Verification items for the finished model (mm, model axes). Face numbers are marked on the shaded views. A direction names the side the tool comes from. Give positions to 0.01 mm unless a question says otherwise; leave off trailing zeros. Loops run counter-clockwise (first coordinate to the right, second up) from the corner with the lowest first, then second, coordinate; pieces in that order, holes last. Notation, with made-up numbers: (16, -32) - (72, -32) arc R5 cw to (72, -25) - close; hole circle Ø4 at (4, 14.5). An arc over 180 degrees is marked (long way). One line per question, with ' | ' between items. Start each with the question number.
1. Thickness scan on line 1 along Y through (x, z) = (24, 34); line 2 along X through (y, z) = (109.25, 5); line 3 along Y through (x, z) = (4, 23.5). Record the ranges inside material, lowest first. Write a range as from..to.
2. Section check A-A, the plane z = 19.5. State how many separate pieces and enclosed holes the cut face has, then the cut area to 3 significant figures.
3. Depth check by flat-ended pin: pin 1 Ø6.5 at (x, y) = (58, 3) entering from -Z; pin 2 Ø10 at (x, y) = (10.5, 77) entering from -Z; pin 3 Ø1.3 at (x, y) = (59, 109) entering from +Z; pin 4 Ø2 at (x, y) = (46.5, 67) entering from +Z. Enter the tip coordinate at first touch or a pass-through.
4. Tool access check on the marked faces 5, 6 and 7. Record the directions out of +Z, -Z, +X, -X, +Y, -Y that give a thin tool (end or side, any length) a straight path to the whole face; none if there is none.
5. Mould release check, pull along X, two halves, no side actions. Record for the marked faces 1, 2, 3 and 4: +X half, -X half, draft (parallel to the pull), parting line (faces both ways), or undercut.
6. Section check B-B, the plane y = 28. Enter the section's corners in (x, z), then the cut area to 3 significant figures.
7. Section check C-C, the plane z = 9. Enter the section's corners in (x, y).
8. Section check D-D, the plane y = 63.5. Enter the section's corners in (x, z), then the cut area to 3 significant figures.
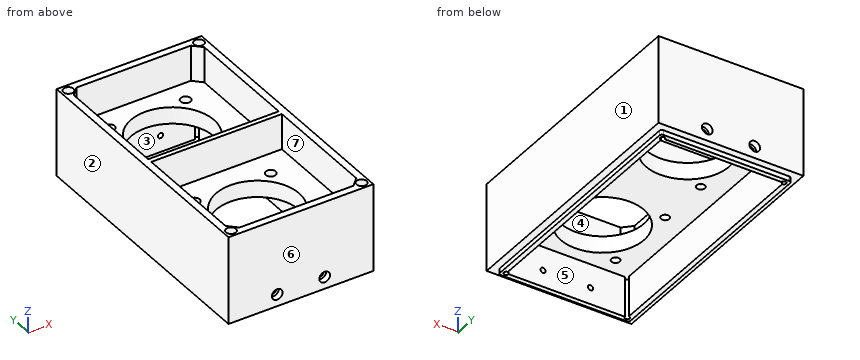
from build123d import *

# Parameters (mm, degrees)
SKETCH1_W           = 61
SKETCH1_H           = 111
SKETCH1_W_2         = 51
SKETCH1_H_2         = 101
BOSS_EXTRUDE1_DEPTH = 15
SKETCH2_W           = 61
SKETCH2_H           = 111
BOSS_EXTRUDE2_DEPTH = 7
SKETCH3_R           = 17.5
SKETCH3_R_2         = 1.75
CUT_EXTRUDE1_DEPTH  = 23
SKETCH4_R           = 2.1
CUT_EXTRUDE2_DEPTH  = 5
SKETCH5_W           = 55
SKETCH5_H           = 105
SKETCH5_W_2         = 51
SKETCH5_H_2         = 101
BOSS_EXTRUDE3_DEPTH = 2
FILLET1_R           = 1
SKETCH6_R           = 1.1
CUT_EXTRUDE3_DEPTH  = 112
SKETCH7_R           = 2.25
CUT_EXTRUDE4_DEPTH  = 2.5
SKETCH8_R           = 2.25
CUT_EXTRUDE5_DEPTH  = 2.5
CUT_EXTRUDE6_START  = -17
SKETCH9_R           = 1
CUT_EXTRUDE6_DEPTH  = 17
SKETCH10_W          = 61
SKETCH10_H          = 111
SKETCH10_W_2        = 55
SKETCH10_H_2        = 105
SKETCH10_H_3        = 2
BOSS_EXTRUDE4_DEPTH = 15
SKETCH11_R          = 2.1
CUT_EXTRUDE7_DEPTH  = 6


with BuildPart() as part:
    # Sketch1 → Boss-Extrude1 (new body)
    with BuildSketch(Plane.XY):
        with Locations((30.5, 55.5)):
            Rectangle(SKETCH1_W, SKETCH1_H)
        with Locations((30.5, 55.5)):
            Rectangle(SKETCH1_W_2, SKETCH1_H_2, mode=Mode.SUBTRACT)
    extrude(amount=BOSS_EXTRUDE1_DEPTH)

    # Sketch2 → Boss-Extrude2 (add)
    with BuildSketch(Plane.XY.offset(15)):
        with Locations((30.5, 55.5)):
            Rectangle(SKETCH2_W, SKETCH2_H)
    extrude(amount=BOSS_EXTRUDE2_DEPTH)

    # Sketch3 → Cut-Extrude1 (cut, through all)
    with BuildSketch(Plane.XY.offset(22)):
        with Locations((30.5, 83)):
            Circle(SKETCH3_R)
        with Locations((30.5, 28)):
            Circle(SKETCH3_R)
        with BuildLine():
            ThreePointArc((46.5, 13.75), (45.262563133, 13.237436867), (44.75, 12))
            Line((44.75, 12), (46.5, 12))
            Line((46.5, 12), (46.5, 13.75))
        make_face()
        with BuildLine():
            Line((46.5, 12), (44.75, 12))
            ThreePointArc((44.75, 12), (46.5, 10.25), (48.25, 12))
            ThreePointArc((48.25, 12), (47.737436867, 13.237436867), (46.5, 13.75))
            Line((46.5, 13.75), (46.5, 12))
        make_face()
        with Locations((46.5, 99)):
            Circle(SKETCH3_R_2)
        with Locations((14.5, 99)):
            Circle(SKETCH3_R_2)
        with Locations((14.5, 67)):
            Circle(SKETCH3_R_2)
        with Locations((46.5, 67)):
            Circle(SKETCH3_R_2)
        with Locations((46.5, 44)):
            Circle(SKETCH3_R_2)
        with Locations((14.5, 44)):
            Circle(SKETCH3_R_2)
        with Locations((14.5, 12)):
            Circle(SKETCH3_R_2)
    extrude(amount=-CUT_EXTRUDE1_DEPTH, mode=Mode.SUBTRACT)

    # Sketch4 → Cut-Extrude2 (cut)
    with BuildSketch(Plane.XY.offset(22)):
        with Locations((14.5, 99)):
            Circle(SKETCH4_R)
        with Locations((46.5, 99)):
            Circle(SKETCH4_R)
        with Locations((46.5, 67)):
            Circle(SKETCH4_R)
        with Locations((46.5, 44)):
            Circle(SKETCH4_R)
        with Locations((14.5, 67)):
            Circle(SKETCH4_R)
        with Locations((14.5, 44)):
            Circle(SKETCH4_R)
        with Locations((14.5, 12)):
            Circle(SKETCH4_R)
        with Locations((46.5, 12)):
            Circle(SKETCH4_R)
    extrude(amount=-CUT_EXTRUDE2_DEPTH, mode=Mode.SUBTRACT)

    # Sketch5 → Boss-Extrude3 (add)
    with BuildSketch(Plane(origin=(0, 0, 0), x_dir=(-1, 0, 0), z_dir=(0, 0, -1))):
        with Locations((-30.5, 55.5)):
            Rectangle(SKETCH5_W, SKETCH5_H)
        with Locations((-30.5, 55.5)):
            Rectangle(SKETCH5_W_2, SKETCH5_H_2, mode=Mode.SUBTRACT)
    extrude(amount=BOSS_EXTRUDE3_DEPTH)

    # Fillet1
    fillet1_edges = [part.edges().sort_by_distance(p)[0] for p in [
        (58, 3, -1),
        (3, 3, -1),
        (3, 108, -1),
        (58, 108, -1),
    ]]
    fillet(fillet1_edges, radius=FILLET1_R)

    # Sketch6 → Cut-Extrude3 (cut, through all)
    with BuildSketch(Plane(origin=(0, 0, 0), x_dir=(-1, 0, 0), z_dir=(0, -1, 0))):
        with Locations((-20.5, -5)):
            Circle(SKETCH6_R)
        with Locations((-40.5, -5)):
            Circle(SKETCH6_R)
    extrude(amount=-CUT_EXTRUDE3_DEPTH, mode=Mode.SUBTRACT)

    # Sketch7 → Cut-Extrude4 (cut)
    with BuildSketch(Plane.XZ):
        with Locations((20.5, 5)):
            Circle(SKETCH7_R)
        with Locations((40.5, 5)):
            Circle(SKETCH7_R)
    extrude(amount=-CUT_EXTRUDE4_DEPTH, mode=Mode.SUBTRACT)

    # Sketch8 → Cut-Extrude5 (cut)
    with BuildSketch(Plane(origin=(0, 111, 0), x_dir=(1, 0, 0), z_dir=(0, 1, 0))):
        with Locations((40.5, -5)):
            Circle(SKETCH8_R)
        with Locations((20.5, -5)):
            Circle(SKETCH8_R)
    extrude(amount=-CUT_EXTRUDE5_DEPTH, mode=Mode.SUBTRACT)

    # Sketch9 → Cut-Extrude6 (cut)
    with BuildSketch(Plane(origin=(0, 0, -2), x_dir=(-1, 0, 0), z_dir=(0, 0, -1)).offset(CUT_EXTRUDE6_START)):
        with Locations((-56, 106)):
            Circle(SKETCH9_R)
        with Locations((-5, 106)):
            Circle(SKETCH9_R)
        with Locations((-5, 5)):
            Circle(SKETCH9_R)
        with Locations((-56, 5)):
            Circle(SKETCH9_R)
    extrude(amount=CUT_EXTRUDE6_DEPTH, mode=Mode.SUBTRACT)

    # Sketch10 → Boss-Extrude4 (add)
    with BuildSketch(Plane.XY.offset(22)):
        with Locations((30.5, 55.5)):
            Rectangle(SKETCH10_W, SKETCH10_H)
        with Locations((30.5, 55.5)):
            Rectangle(SKETCH10_W_2, SKETCH10_H_2, mode=Mode.SUBTRACT)
        Polygon((3, 3), (6.535533906, 3), (3, 6.535533906), align=None)
        Polygon((3, 108), (3, 104.58049017), (6.41950983, 108), align=None)
        Polygon((54.58049017, 108), (58, 104.58049017), (58, 108), align=None)
        Polygon((58, 6.41950983), (54.58049017, 3), (58, 3), align=None)
        with Locations((30.5, 55.5)):
            Rectangle(SKETCH10_W_2, SKETCH10_H_3)
    extrude(amount=BOSS_EXTRUDE4_DEPTH)

    # Sketch11 → Cut-Extrude7 (cut)
    with BuildSketch(Plane.XY.offset(37)):
        with Locations((3, 3)):
            Circle(SKETCH11_R)
        with Locations((3, 108)):
            Circle(SKETCH11_R)
        with Locations((58, 108)):
            Circle(SKETCH11_R)
        with Locations((58, 3)):
            Circle(SKETCH11_R)
    extrude(amount=-CUT_EXTRUDE7_DEPTH, mode=Mode.SUBTRACT)


solid = part.part
Results list:
1) line 1: 0..3, 54.5..56.5, 108..111 | line 2: 0..18.25, 22.75..38.25, 42.75..61 | line 3: 0..5.54, 54.5..56.5, 105.58..111
2) separate pieces: 1 | enclosed holes: 10 | area: 4,740 mm²
3) pin 1: z = -2 | pin 2: z = 15 | pin 3: z = 31 | pin 4: through
4) face 5: -Z | face 6: +Z, -Z, +X, -X, -Y | face 7: +Z
5) face 1: +X half | face 2: -X half | face 3: undercut | face 4: undercut
6) outline: (0, 0) - (3, 0) - (3, -2) - (5, -2) - (5, 15) - (13, 15) - (13, 22) - (3, 22) - (3, 37) - (0, 37) - close; (48, 15) - (56, 15) - (56, -2) - (58, -2) - (58, 0) - (61, 0) - (61, 37) - (58, 37) - (58, 22) - (48, 22) - close | area: 430 mm²
7) outline: (0, 0) - (61, 0) - (61, 111) - (0, 111) - close; hole (5, 6) arc R1 ccw (long way) to (6, 5) - (55, 5) arc R1 ccw (long way) to (56, 6) - (56, 105) arc R1 ccw (long way) to (55, 106) - (6, 106) arc R1 ccw (long way) to (5, 105) - close
8) outline: (0, 0) - (3, 0) - (3, -2) - (5, -2) - (5, 15) - (56, 15) - (56, -2) - (58, -2) - (58, 0) - (61, 0) - (61, 37) - (58, 37) - (58, 22) - (3, 22) - (3, 37) - (0, 37) - close | area: 675 mm²
